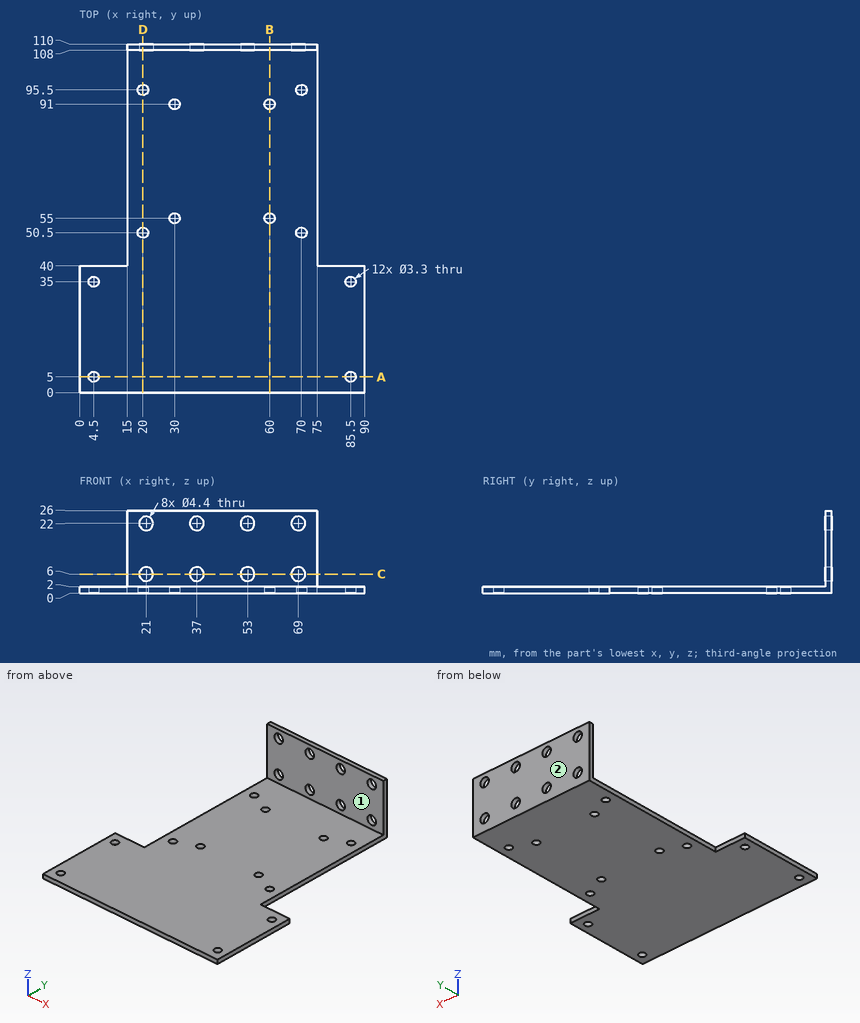
Geometry: see drawing. Coordinates: mm, zero at the bounding-box minimum. A direction names the side the tool comes from. Round coordinates to 2 decimals unless told otherwise and drop trailing zeros. Loops run counter-clockwise (first coordinate to the right, second up) from the corner with the lowest first, then second, coordinate; pieces in that order, holes last. Notation, with made-up numbers: (78.5, -30) - (109.5, -30) arc R8 cw to (109.5, -19) - close; hole circle Ø4 at (26.25, 55.5). An arc over 180 degrees is marked (long way). Write item = value, one per line. Start each with the question number.
(1) Section query A-A, the plane y = 5. Output: boundary loops of the cut face in (x, z).
(2) Set-up query: the marked faces 1 and 2. Return all of +Z, -Z, +X, -X, +Y, -Y with unobstructed straight access to the full face (end or side cutting, diameter ignored); none if empty.
(3) Ray query, line 1 along Y through (x, z) = (30, 0.75); line 2 along Y through (x, z) = (85.5, 0.6); line 3 along Z through (x, y) = (21, 109.35). Return the intervals inside material, ascending. Write a range as from..to.
(4) Section query D-D, the plane x = 20. Output: boundary loops of the cut face in (y, z), plus the area to 3 significant figures.
(5) Section query B-B, the plane x = 60. Output: boundary loops of the cut face in (y, z).
(6) Pin query (flat end, axial travel): pin 1 (2 mm diameter, centred on x = 81.5, z = 1, fed in from +Y); pin 2 (4 mm diameter, centred on x = 74.5, y = 59.5, fed in from +Z); pin 3 (7 mm diameter, centred on x = 69, z = 6, fed in from -Y). Return the tip coordinate at first contact, or that it passes through.
(7) Section query C-C, the plane z = 6. Output: boundary loops of the cut face in (x, y), plus the area to 3 significant figures.
Conclusion:
q1.outline = (0, 0) - (2.85, 0) - (2.85, 2) - (0, 2) - close; (6.15, 0) - (83.85, 0) - (83.85, 2) - (6.15, 2) - close; (87.15, 0) - (90, 0) - (90, 2) - (87.15, 2) - close
q2.face_1 = +Z, +X, -X, -Y
q2.face_2 = +Z, -Z, +X, -X, +Y
q3.line_1 = 0..53.35, 56.65..89.35, 92.65..110
q3.line_2 = 0..3.35, 6.65..33.35, 36.65..40
q3.line_3 = 0..3.8, 8.2..19.8, 24.2..26
q4.outline = (0, 0) - (48.85, 0) - (48.85, 2) - (0, 2) - close; (52.15, 0) - (93.85, 0) - (93.85, 2) - (52.15, 2) - close; (97.15, 0) - (110, 0) - (110, 4.04) - (108, 4.04) - (108, 2) - (97.15, 2) - close; (108, 7.96) - (110, 7.96) - (110, 20.04) - (108, 20.04) - close; (108, 23.96) - (110, 23.96) - (110, 26) - (108, 26) - close
q4.area = 239 mm2
q5.outline = (0, 0) - (53.35, 0) - (53.35, 2) - (0, 2) - close; (56.65, 0) - (89.35, 0) - (89.35, 2) - (56.65, 2) - close; (92.65, 0) - (110, 0) - (110, 26) - (108, 26) - (108, 2) - (92.65, 2) - close
q6.pin_1 = 40
q6.pin_2 = 2
q6.pin_3 = 108
q7.outline = (15, 108) - (18.8, 108) - (18.8, 110) - (15, 110) - close; (23.2, 108) - (34.8, 108) - (34.8, 110) - (23.2, 110) - close; (39.2, 108) - (50.8, 108) - (50.8, 110) - (39.2, 110) - close; (55.2, 108) - (66.8, 108) - (66.8, 110) - (55.2, 110) - close; (71.2, 108) - (75, 108) - (75, 110) - (71.2, 110) - close
q7.area = 84.8 mm2
